Print and shaded views of the part. All mm, measured from the part's lowest x, y and z. A direction names the side the tool comes from. Coordinates: 2 decimals unless noted, no trailing zeros. Order: outer loops, then holes, each group sorted by start corner. A loop starts at its lowest first (then second) coordinate and runs counter-clockwise, first axis right, second up. Notation, with made-up numbers: (77.25, 43.25) -> (101.25, 43.25) arc R33 cw to (101.25, 74.25) -> close; hole circle Ø1 at (-2.5, -27). An arc over 180 degrees is marked (long way). Write item = value, one per line. Start each with the question number.
Q1. Mould opens along X. For the marked faces 3, 4, 5 and 6 say: +X half, -X half, draft (parallel to the pull), parting line (faces both ways), or undercut.
Q2. Flat gauge pins, fed straight in: pin 1 (2 mm diameter, centred on x = 12.5, z = 2.5, fed in from -Y); pin 2 (3 mm diameter, centred on x = 22.5, y = 26.38, fed in from -Z). Where does each tip first touch, or does it go through?
Q3. Cut at C-C, the plane y = 2.5. List the corners of the cut face in (x, z), plus the area to 3 significant figures.
Q4. Cut at D-D, the plane z = 2.8. List the corners of the cut face in (x, y).
Q5. 3-axis set-ups, long thin cutter, end or side, ignore diameter. For the marked faces 1 and 2: which of +Z, -Z, +X, -X, +Y, -Y reach the whole face in a straight line?
Q6. Wall check: line 1 (Y direction, x = 22.5, z = 0.8) (1 decimal); line 2 (X direction, y = 12, z = 0.3); line 3 (Y direction, x = 21, z = 3.55) (1 decimal). Give the ranges that are in metal, low to high. Write a range as from..to.
Q7. Cut at B-B, the plane y = 18. List the corners of the cut face in (x, z), plus the area to 3 significant figures.
Q8. Cut at A-A, the plane x = 2.5. List the corners of the cut face in (y, z).
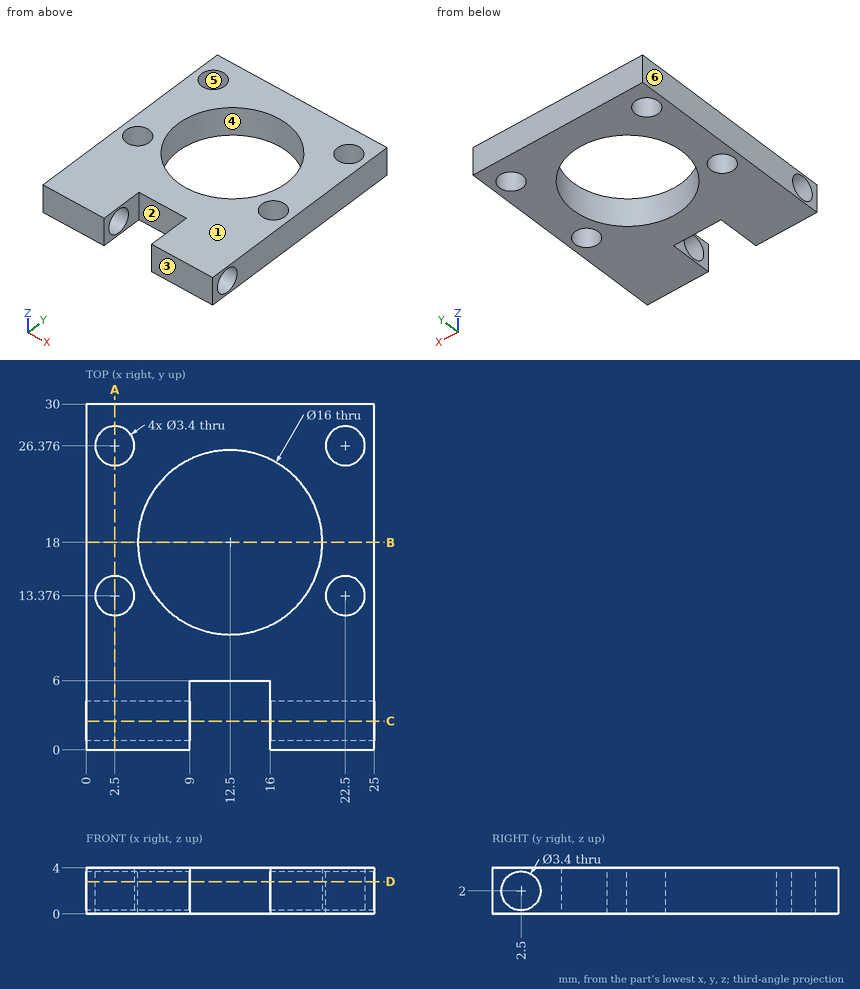
Here are the results:
q1.face_3 = draft
q1.face_4 = undercut
q1.face_5 = undercut
q1.face_6 = -X half
q2.pin_1 = 6
q2.pin_2 = through
q3.outline = (0, 0) -> (9, 0) -> (9, 0.3) -> (0, 0.3) -> close; (0, 3.7) -> (9, 3.7) -> (9, 4) -> (0, 4) -> close; (16, 0) -> (25, 0) -> (25, 0.3) -> (16, 0.3) -> close; (16, 3.7) -> (25, 3.7) -> (25, 4) -> (16, 4) -> close
q3.area = 10.8 mm²
q4.outline = (0, 0) -> (9, 0) -> (9, 1) -> (0, 1) -> close; (0, 4) -> (9, 4) -> (9, 6) -> (16, 6) -> (16, 4) -> (25, 4) -> (25, 30) -> (0, 30) -> close; (16, 0) -> (25, 0) -> (25, 1) -> (16, 1) -> close; hole circle Ø3.4 at (2.5, 13.38); hole circle Ø3.4 at (2.5, 26.38); hole circle Ø16 at (12.5, 18); hole circle Ø3.4 at (22.5, 13.38); hole circle Ø3.4 at (22.5, 26.38)
q5.face_1 = +Z, +X, -X, +Y, -Y
q5.face_2 = +Z, -Z, -Y
q6.line_1 = 0..1.3, 3.7..11.7, 15.1..24.7, 28.1..30
q6.line_2 = 0..1.5, 3.5..7.21, 17.79..21.5, 23.5..25
q6.line_3 = 0..1.8, 3.2..12.6, 14.2..25.6, 27.2..30
q7.outline = (0, 0) -> (4.5, 0) -> (4.5, 4) -> (0, 4) -> close; (20.5, 0) -> (25, 0) -> (25, 4) -> (20.5, 4) -> close
q7.area = 36.0 mm²
q8.outline = (0, 0) -> (11.68, 0) -> (11.68, 4) -> (0, 4) -> close; (15.08, 0) -> (24.68, 0) -> (24.68, 4) -> (15.08, 4) -> close; (28.08, 0) -> (30, 0) -> (30, 4) -> (28.08, 4) -> close; hole circle Ø3.4 at (2.5, 2)
